Design review of the part built by this model. Coordinates are the model's own, in mm. A direction names the side the tool comes from. Coordinates: 2 decimals unless noted, no trailing zeros. Write each loop counter-clockwise with the first axis right and the second up, starting at its lowest first coordinate (ties: lowest second). Pieces come first, ordered by that corner, then holes. Notation, with made-up numbers: (41.25, -22.5) - (62.25, -22.5) arc R20 ccw to (62.25, 9.5) - close; hole circle Ø5 at (43, -37). An arc over 180 degrees is marked (long way). Answer as a JSON object with one key per item and string values.
```python
from build123d import *

# Parameters (mm, degrees)
BOSS_EXTRUDE1_DEPTH     = 18
FILLET1_R               = 40
FILLET2_R               = 10
CUT_EXTRUDE1_DEPTH      = 75.41915473
CUT_EXTRUDE1_DEPTH_BACK = 75.41915473
SKETCH8_R               = 1.52
FILLET3_R               = 5
SKETCH13_R              = 1.625
CUT_EXTRUDE6_DEPTH      = 10
SKETCH14_R              = 1.625
CUT_EXTRUDE7_DEPTH      = 10


with BuildPart() as part:
    # Sketch7 → Boss-Extrude1 (new body)
    with BuildSketch(Plane(origin=(0, 0, 0), x_dir=(1, 0, 0), z_dir=(0, 1, 0))):
        with BuildLine():
            Line((3.5, 0), (18.2, 0))
            Line((18.2, 0), (20.800813361, 4.113644998))
            ThreePointArc((20.800813361, 4.113644998), (21.592172613, 7.217756586), (23.7, 9.629980027))
            Line((23.7, 9.629980027), (23.7, 23.144126484))
            Line((23.7, 23.144126484), (26.2, 23.144126484))
            Line((26.2, 23.144126484), (26.2, 8.144126484))
            ThreePointArc((26.2, 8.144126484), (27.7, -0.392297092), (29.2, 8.144126484))
            Line((29.2, 8.144126484), (29.2, 23.144126484))
            Line((29.2, 23.144126484), (31.7, 23.144126484))
            Line((31.7, 23.144126484), (31.7, 9.629980027))
            ThreePointArc((31.7, 9.629980027), (33.807827387, 7.217756586), (34.599186639, 4.113644998))
            Line((34.599186639, 4.113644998), (37.2, 0))
            Line((37.2, 0), (39.2, 0))
            Line((39.2, 0), (39.2, -10))
            Line((39.2, -10), (0, -10))
            Line((0, -10), (0, -2.2))
            Line((0, -2.2), (3.5, 0))
        make_face()
    boss_extrude1 = extrude(amount=BOSS_EXTRUDE1_DEPTH)

    # Mirror1: Boss-Extrude1 across plane
    add(boss_extrude1.mirror(Plane(origin=(0, 18, 10), x_dir=(0, 0, 1), z_dir=(1, 0, 0))))

    # Fillet1
    # the kernel refuses this fillet: 40 mm, written as the material it adds along each edge
    with BuildSketch(Plane(origin=(23.7, 0, -9.629980027), x_dir=(0, 0, -1), z_dir=(0, 1, 0)), Plane(origin=(-31.7, 0, -9.629980027), x_dir=(0, 0, -1), z_dir=(0, 1, 0))) as fillet1_piece_1:
        with BuildLine():
            CenterArc((10.613793835, 40), FILLET1_R, 249.745857862, 20.254142138)
            Line((-3.233601435, 2.473347548), (-3.51054934, 1.722814499))
            ThreePointArc((-3.51054934, 1.722814499), (-1.916270335, 0.845153632), (-0.651858217, -0.463768116))
            Line((-0.651858217, -0.463768116), (0, -0.8))
            Line((0, -0.8), (10.613793835, -0.8))
            Line((10.613793835, -0.8), (10.613793835, 0))
        make_face()
    extrude(amount=18)
    with BuildSketch(Plane(origin=(20.800813361, 0, -4.113644998), x_dir=(0.18333937231858005, 0, -0.9830496806152929), z_dir=(0, 1, 0)), Plane(origin=(-34.599186639, 0, -4.113644998), x_dir=(0.18333937231857603, 0, -0.9830496806152935), z_dir=(0, 1, 0))) as fillet1_piece_2:
        with BuildLine():
            CenterArc((9.050455959, 39.429951175), FILLET1_R, 250.166978756, 10.14844141)
            Line((-4.52074889, 1.802535653), (-4.792172987, 1.049987342))
            ThreePointArc((-4.792172987, 1.049987342), (-2.556670036, 0.158160214), (-0.296295591, -0.743107612))
            Line((-0.296295591, -0.743107612), (0.134579271, -0.788599024))
            ThreePointArc((0.134579271, -0.788599024), (1.16074621, -0.701666578), (2.18691315, -0.788599024))
            Line((2.18691315, -0.788599024), (2.321492421, 0))
        make_face()
    extrude(amount=18)
    with BuildSketch(Plane(origin=(31.7, 0, -9.629980027), x_dir=(0, 0, -1), z_dir=(0, 1, 0))) as fillet1_piece_3:
        with BuildLine():
            CenterArc((10.613793835, -40), FILLET1_R, 90, 20.254142138)
            Line((-3.233601435, -2.473347548), (-3.51054934, -1.722814499))
            ThreePointArc((-3.51054934, -1.722814499), (-1.916270335, -0.845153632), (-0.651858217, 0.463768116))
            Line((-0.651858217, 0.463768116), (0, 0.8))
            Line((0, 0.8), (10.613793835, 0.8))
            Line((10.613793835, 0.8), (10.613793835, 0))
        make_face()
    extrude(amount=18)
    with BuildSketch(Plane(origin=(34.599186639, 0, -4.113644998), x_dir=(0.5343927114747591, 0, 0.8452363160221257), z_dir=(0, 1, 0)), Plane(origin=(-20.800813361, 0, -4.113644998), x_dir=(0.5343927114747586, 0, 0.8452363160221262), z_dir=(0, 1, 0))) as fillet1_piece_4:
        with BuildLine():
            CenterArc((6.196822464, 39.977883812), FILLET1_R, 257.946173426, 10.14844141)
            Line((-2.156398361, 0.859809961), (-2.323462777, 0.077448484))
            ThreePointArc((-2.323462777, 0.077448484), (-1.338075072, -0.221862238), (-0.417081618, -0.682673366))
            Line((-0.417081618, -0.682673366), (0, -0.8))
            ThreePointArc((0, -0.8), (2.433428924, -0.8), (4.840258555, -0.799557676))
            Line((4.840258555, -0.799557676), (4.866857847, 0))
        make_face()
    extrude(amount=18)
    with BuildSketch(Plane(origin=(-23.7, 0, -9.629980027), x_dir=(0.6075420957696648, 0, 0.7942874806188269), z_dir=(0, 1, 0))) as fillet1_piece_5:
        with BuildLine():
            CenterArc((15.871280266, 38.219825775), FILLET1_R, 232.588008111, 20.254142138)
            Line((-8.430403565, 6.44832655), (-8.916437241, 5.812896566))
            Line((-8.916437241, 5.812896566), (-0.486033677, -0.635429984))
            Line((-0.486033677, -0.635429984), (0.236004168, -0.764396516))
            ThreePointArc((0.236004168, -0.764396516), (2.035535945, -0.492919946), (3.835067722, -0.764396516))
            Line((3.835067722, -0.764396516), (4.07107189, 0))
        make_face()
    extrude(amount=18)

    # Fillet2
    # the kernel refuses this fillet: 10 mm, written as the material it takes off along each edge
    with BuildSketch(Plane(origin=(-39.2, -15, 0), x_dir=(1, 0, 0), z_dir=(0, 1, 0))) as fillet2_piece_1:
        with BuildLine():
            CenterArc((10, -6), FILLET2_R, 143.130102354, 36.869897646)
            Line((0, -6), (-0.2, -6))
            Line((-0.2, -6), (-0.2, 0))
            Line((-0.2, 0), (0, 0.2))
            ThreePointArc((0, 0.2), (1, 0.2), (1.84, 0.12))
            Line((1.84, 0.12), (2, 0))
        make_face()
    extrude(amount=48, mode=Mode.SUBTRACT)
    with BuildSketch(Plane(origin=(39.2, -15, 0), x_dir=(0, 0, 1), z_dir=(0, 1, 0))) as fillet2_piece_2:
        with BuildLine():
            CenterArc((6, -10), FILLET2_R, 90, 36.869897646)
            Line((0, -2), (-0.12, -1.84))
            ThreePointArc((-0.12, -1.84), (-0.2, -1), (-0.2, 0))
            Line((-0.2, 0), (0, 0.2))
            Line((0, 0.2), (6, 0.2))
            Line((6, 0.2), (6, 0))
        make_face()
    extrude(amount=48, mode=Mode.SUBTRACT)

    # Sketch8 → Cut-Extrude1 (cut, two sides: drawn at the far end of the back side and taken through both)
    with BuildSketch(Plane.ZY.offset(-29.2).offset(-CUT_EXTRUDE1_DEPTH_BACK)):
        with Locations((-13.144126484, 8.1)):
            Circle(SKETCH8_R)
    extrude(amount=CUT_EXTRUDE1_DEPTH + CUT_EXTRUDE1_DEPTH_BACK, mode=Mode.SUBTRACT)

    # Fillet3
    fillet3_edges = [part.edges().sort_by_distance(p)[0] for p in [
        (0, 9, 2.2),
    ]]
    fillet(fillet3_edges, radius=FILLET3_R)

    # Sketch13 → Cut-Extrude6 (cut)
    with BuildSketch(Plane.XY.offset(10)):
        with Locations((12.725, 3.675)):
            Circle(SKETCH13_R)
        with Locations((34.925, 14.225)):
            Circle(SKETCH13_R)
    extrude(amount=-CUT_EXTRUDE6_DEPTH, mode=Mode.SUBTRACT)

    # Sketch14 → Cut-Extrude7 (cut)
    with BuildSketch(Plane.XY.offset(10)):
        with Locations((12.725, 14.325)):
            Circle(SKETCH14_R)
        with Locations((34.925, 3.775)):
            Circle(SKETCH14_R)
    extrude(amount=-CUT_EXTRUDE7_DEPTH, mode=Mode.SUBTRACT)


solid = part.part
```
(1) Take a section at B-B, the plane y = 8.1. Give the number of separate pieces and of enclosed holes in the cut face, and give its area (3 significant figures).
Solved:
{"separate pieces": "5", "enclosed holes": "0", "area": "1,040 mm^2"}
(2) For pin 1 (8 mm diameter, centred on y = 14.5, z = -14, fed in from -X); pin 2 (3 mm diameter, centred on y = 10.5, z = -22, fed in from -X); pin 3 (4 mm diameter, centred on y = 11, z = 3, fed in from -X), all flat-tipped, find the tip position at first contact; note any pin that passes through.
Solved:
{"pin 1": "stops at x = -33.03", "pin 2": "stops at x = -31.7", "pin 3": "stops at x = -39.15"}
(3) To check wall thickness, follow line 1 (X direction, y = 6.75, z = -19); line 2 (X direction, y = 4.5, z = 4) (3 decimals); line 3 (X direction, y = 4.5, z = -7.5). State the ranges of each line that lie inside material, in increasing order. Write a range as from..to.
Solved:
{"line 1": "x = -31.72..-29.2, -26.2..-23.68, 23.68..26.2, 29.2..31.72", "line 2": "x = -38.998..11.325, 14.125..33.471, 36.379..38.998", "line 3": "x = -33.78..-30.38, -25.02..-21.62, 21.62..25.02, 30.38..33.78"}
(4) Take a section at A-A, the plane z = -10. Write out the cut boundary in (x, y), and give its area (3 significant figures).
Solved:
{"outline": "(-33.03, 0) - (-29.2, 0) - (-29.2, 18) - (-33.03, 18) - close; (-26.2, 0) - (-22.37, 0) - (-22.37, 18) - (-26.2, 18) - close; (22.37, 0) - (26.2, 0) - (26.2, 18) - (22.37, 18) - close; (29.2, 0) - (33.03, 0) - (33.03, 18) - (29.2, 18) - close", "area": "276 mm^2"}
(5) Take a section at C-C, the plane z = 2. Write out the cut boundary in (x, y) (3 decimals), and give its area (3 significant figures).
Solved:
{"outline": "(-38.365, 0) - (38.365, 0) - (38.365, 18) - (-38.365, 18) - close; hole circle Ø3.25 at (12.725, 3.675); hole circle Ø3.25 at (12.725, 14.325); hole circle Ø3.25 at (34.925, 3.775); hole circle Ø3.25 at (34.925, 14.225)", "area": "1,350 mm^2"}
(6) Take a section at D-D, the plane x = 19.5. Write out the cut boundary in (y, z).
Solved:
{"outline": "(0, -2.4) - (18, -2.4) - (18, 10) - (0, 10) - close"}
(7) Tool access review of faces 3 (the face through (31.7, 9, -22)), 4 (the face through (-11, 9, 0)), 5 (the face through (36.475, 14.713, 5.07)): name each direction out of +Z, -Z, +X, -X, +Y, -Y from which nothing blocks a thin tool from reaching the whole face with its end or side.
Solved:
{"face 3": "-Z, +X, +Y, -Y", "face 4": "-Z, +Y, -Y", "face 5": "+Z"}
(8) The part is to be moulded in two halves that separate along Y. For faces 1 (the face through (-23.7, 9, -22)), 2 (the face through (-24.456, 8.557, -11.694)), say which applies: pulls with the +Y half, pulls with the -Y half, needs draft (parallel to the pull), parting line crosses it, or undercut.
Solved:
{"face 1": "needs draft", "face 2": "undercut"}
